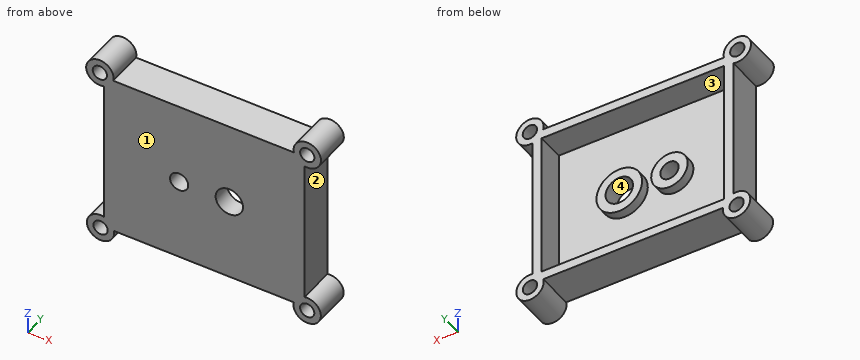
```python
from build123d import *

# Parameters (mm, degrees)
SKETCH1_W           = 69.85
SKETCH1_H           = 57.15
BOSS_EXTRUDE1_DEPTH = 12.7
SKETCH2_W           = 63.5
SKETCH2_H           = 50.8
CUT_EXTRUDE1_DEPTH  = 9.525
SKETCH3_R           = 6.35
SKETCH3_R_2         = 3.175
SKETCH3_R_3         = 7.9375
SKETCH3_R_4         = 4.7625
BOSS_EXTRUDE2_DEPTH = 3.175
SKETCH5_R           = 3.175
CUT_EXTRUDE2_DEPTH  = 46.5698228
SKETCH6_R           = 4.7625
CUT_EXTRUDE3_DEPTH  = 46.5698228
SKETCH8_R           = 4.7625
BOSS_EXTRUDE3_DEPTH = 12.7
SKETCH9_R           = 2.4892
CUT_EXTRUDE4_DEPTH  = 56.068582541


with BuildPart() as part:
    # Sketch1 → Boss-Extrude1 (new body)
    with BuildSketch(Plane(origin=(0, 0, 0), x_dir=(1, 0, 0), z_dir=(0, 1, 0))):
        Rectangle(SKETCH1_W, SKETCH1_H)
    extrude(amount=BOSS_EXTRUDE1_DEPTH)

    # Sketch2 → Cut-Extrude1 (cut)
    with BuildSketch(Plane(origin=(0, 12.7, 0), x_dir=(1, 0, 0), z_dir=(0, 1, 0))):
        Rectangle(SKETCH2_W, SKETCH2_H)
    extrude(amount=-CUT_EXTRUDE1_DEPTH, mode=Mode.SUBTRACT)

    # Sketch3 → Boss-Extrude2 (add)
    # profile 1 of 2: a face of its own
    with BuildSketch(Plane(origin=(0, 3.175, 0), x_dir=(1, 0, 0), z_dir=(0, 1, 0))):
        with Locations(Location((-8.73125, 0, 0), (0, 0, 90))):
            Circle(SKETCH3_R)
        with Locations(Location((-8.73125, 0, 0), (0, 0, 270))):
            Circle(SKETCH3_R_2, mode=Mode.SUBTRACT)
    # profile 2 of 2: a face of its own
    with BuildSketch(Plane(origin=(0, 3.175, 0), x_dir=(1, 0, 0), z_dir=(0, 1, 0))):
        with Locations(Location((8.73125, 0, 0), (0, 0, 90))):
            Circle(SKETCH3_R_3)
        with Locations(Location((8.73125, 0, 0), (0, 0, 270))):
            Circle(SKETCH3_R_4, mode=Mode.SUBTRACT)
    extrude(amount=BOSS_EXTRUDE2_DEPTH)

    # Sketch5 → Cut-Extrude2 (cut, through all)
    with BuildSketch(Plane(origin=(0, 6.35, 0), x_dir=(1, 0, 0), z_dir=(0, 1, 0))):
        with Locations(Location((-8.73125, 0, 0), (0, 0, 270))):
            Circle(SKETCH5_R)
    extrude(amount=-CUT_EXTRUDE2_DEPTH, mode=Mode.SUBTRACT)

    # Sketch6 → Cut-Extrude3 (cut, through all)
    with BuildSketch(Plane(origin=(0, 6.35, 0), x_dir=(1, 0, 0), z_dir=(0, 1, 0))):
        with Locations(Location((8.73125, 0, 0), (0, 0, 270))):
            Circle(SKETCH6_R)
    extrude(amount=-CUT_EXTRUDE3_DEPTH, mode=Mode.SUBTRACT)

    # Sketch8 → Boss-Extrude3 (add)
    with BuildSketch(Plane(origin=(0, 12.7, 0), x_dir=(1, 0, 0), z_dir=(0, 1, 0))):
        with Locations((-36.080944449, 29.359475258)):
            Circle(SKETCH8_R)
        with Locations((35.832665303, 29.636957013)):
            Circle(SKETCH8_R)
        with Locations((35.864779118, -29.608646076)):
            Circle(SKETCH8_R)
        with Locations((-36.322, -29.590559194)):
            Circle(SKETCH8_R)
    extrude(amount=-BOSS_EXTRUDE3_DEPTH)

    # Sketch9 → Cut-Extrude4 (cut, through all)
    with BuildSketch(Plane(origin=(0, 12.7, 0), x_dir=(1, 0, 0), z_dir=(0, 1, 0))):
        with Locations(Location((-36.080944449, 29.359475258, 0), (0, 0, 270))):
            Circle(SKETCH9_R)
        with Locations(Location((-36.322, -29.590559194, 0), (0, 0, 270))):
            Circle(SKETCH9_R)
        with Locations(Location((35.864779118, -29.608646076, 0), (0, 0, 270))):
            Circle(SKETCH9_R)
        with Locations(Location((35.832665303, 29.636957013, 0), (0, 0, 270))):
            Circle(SKETCH9_R)
    extrude(amount=-CUT_EXTRUDE4_DEPTH, mode=Mode.SUBTRACT)


solid = part.part
```
For this review, take the finished solid that the model builds, in its own axes (mm). Face numbers are marked on the shaded views. A direction names the side the tool comes from. Round coordinates to 2 decimals unless told otherwise and drop trailing zeros. Loops run counter-clockwise (first coordinate to the right, second up) from the corner with the lowest first, then second, coordinate; pieces in that order, holes last.
Q1. Add section B-B on y = 2. Give the number of separate pieces and of enclosed holes in the cut face, plus the area to 3 significant figures.
Result sheet:
separate pieces: 1
enclosed holes: 6
area: 4,060 mm2
Q2. Insertion check: pin 1 Ø6.5 at (y, z) = (4.5, -2) entering from +X (3 decimals); pin 2 Ø5 at (x, z) = (-13.5, 17) entering from +Y (3 decimals); pin 3 Ø2 at (x, y) = (22, 8) entering from -Z (3 decimals); pin 4 Ø3 at (x, z) = (-36.32, 29.59) entering from -Y. Each pin has a flat end and moves straight along its axis. Give the tip position at first contact, or say it passes through.
Result sheet:
pin 1: stops at x = 34.925
pin 2: stops at y = 3.175
pin 3: stops at z = -28.575
pin 4: passes through
Q3. Add section D-D on z = -23.5. Write out the cut boundary in (x, y) (3 decimals), plus the area to 3 significant figures.
Result sheet:
outline: (-34.925, 0) - (34.925, 0) - (34.925, 12.7) - (31.75, 12.7) - (31.75, 3.175) - (-31.75, 3.175) - (-31.75, 12.7) - (-34.925, 12.7) - close
area: 282 mm2
Q4. To check wall thickness, follow line 1 along X through (y, z) = (2, 29.5); line 2 along X through (y, z) = (5, 0) (3 decimals); line 3 along X through (y, z) = (4.25, -14) (3 decimals). State the ranges of each line that lie inside material, in increasing order.
Result sheet:
line 1: x = -41.08 to -38.81, -33.83 to -31.56, 31.1 to 33.38, 38.35 to 40.63
line 2: x = -34.925 to -31.75, -15.081 to -11.906, -5.556 to -2.381, 0.794 to 3.969, 13.494 to 16.669, 31.75 to 34.925
line 3: x = -34.925 to -31.75, 31.75 to 34.925
Q5. Add section A-A on z = 0. Write out the cut boundary in (x, y) (3 decimals).
Result sheet:
outline: (-34.925, 0) - (-11.906, 0) - (-11.906, 6.35) - (-15.081, 6.35) - (-15.081, 3.175) - (-31.75, 3.175) - (-31.75, 12.7) - (-34.925, 12.7) - close; (-5.556, 0) - (3.969, 0) - (3.969, 6.35) - (0.794, 6.35) - (0.794, 3.175) - (-2.381, 3.175) - (-2.381, 6.35) - (-5.556, 6.35) - close; (13.494, 0) - (34.925, 0) - (34.925, 12.7) - (31.75, 12.7) - (31.75, 3.175) - (16.669, 3.175) - (16.669, 6.35) - (13.494, 6.35) - close
Q6. Add section C-C on x = 28.5. Write out the cut boundary in (y, z) (3 decimals), plus the area to 3 significant figures.
Result sheet:
outline: (0, -28.575) - (12.7, -28.575) - (12.7, -25.4) - (3.175, -25.4) - (3.175, 25.4) - (12.7, 25.4) - (12.7, 28.575) - (0, 28.575) - close
area: 242 mm2
Q7. Mouldability with a two-part tool opening along Z and no side actions: class the marked faces 1 and 2 as +Z half, -Z half, draft (parallel to the pull), parting line (faces both ways), or undercut.
Result sheet:
face 1: draft
face 2: undercut
Q8. Machinability: for the marked faces 3 and 4, which of the approach directions +Z, -Z, +X, -X, +Y, -Y give a long, thin tool a straight path to every point of the face, cutting with its end or side? Answer none if there is none.
Result sheet:
face 3: +Y
face 4: +Y, -Y
